Input: part model. Units: mm. Frame: model coordinates. Face numbers are marked on the shaded views. A direction names the side the tool comes from. Give positions to 0.01 mm unless a question says otherwise; leave off trailing zeros. Order: outer loops, then holes, each group sorted by start corner. A loop starts at its lowest first (then second) coordinate and runs counter-clockwise, first axis right, second up. Notation, with made-up numbers: (28, 4) - (67, 4) arc R21 ccw to (67, 28) - close; hole circle Ø9 at (35, 26.5). An arc over 180 degrees is marked (long way). Answer in a Markdown table with one row per item. Add a question column.
1. Mould query, pull axis X, two halves, no side actions, for the marked faces 1, 2, 3 and 4. Classes: released by +X, released by -X, zero draft, split by the parting line, or undercut.
2. Section query B-B on z = 7.5. Return loops of the section in (x, y) (3 decimals).
3. Section query C-C on z = -9. Return loops of the section in (x, y) (1 decimal).
4. Ray query, line 1 (Y direction, x = 17, z = 31); line 2 (X direction, y = -5.25, z = -25.5); line 3 (X direction, y = -3, z = -25). Return the intervals inside material, ascending. Write a range as [from, to].
5. Access query for the marked faces 5 and 6. Directions: +Z, -Z, +X, -X, +Y, -Y. A direction counts if a zero-diameter tool reaches every point of the face in a straight line with its end or side. Return the directions, or none.
6. Section query A-A on x = 12.7. Return loops of the section in (y, z) (1 decimal).
7. Contact query for flat-ended pins moving along their axis: pin 1 (6.5 mm diameter, centred on x = 37, y = -1, fed in from +Z); pin 2 (2 mm diameter, centred on y = -6, z = 27, fed in from +X); pin 3 (5 mm diameter, centred on x = 18.5, z = -7.5, fed in from +Y). Output: stop coordinate, or through.
```python
from build123d import *

# Parameters (mm, degrees)
EXTRUDE_THIN1_DEPTH = 38.1
EXTRUDE_THIN2_START = 12.7
EXTRUDE_THIN2_DEPTH = 12.7
REVOLVE_THIN1_ANGLE = 180
EXTRUDE_THIN3_START = -10.16
EXTRUDE_THIN3_DEPTH = 1.27


# Read off the part's stored shape, not the designer's step: Extrude-Thin3
with BuildPart() as part:
    # Sketch1 → Extrude-Thin1 (new body)
    with BuildSketch(Plane.XY):
        with BuildLine():
            ThreePointArc((-8.798818102, -5.08), (-5.08, -8.798818102), (0, -10.16))
            Line((0, -10.16), (25.4, -10.16))
            ThreePointArc((25.4, -10.16), (30.48, -8.798818102), (34.198818102, -5.08))
            Line((34.198818102, -5.08), (33.09896584, -4.445))
            ThreePointArc((33.09896584, -4.445), (29.845, -7.69896584), (25.4, -8.89))
            Line((25.4, -8.89), (0, -8.89))
            ThreePointArc((0, -8.89), (-4.445, -7.69896584), (-7.69896584, -4.445))
            Line((-7.69896584, -4.445), (-8.798818102, -5.08))
        make_face()
    extrude(amount=EXTRUDE_THIN1_DEPTH)

    # Sketch2 → Extrude-Thin2 (add)
    with BuildSketch(Plane(origin=(0, 0, 0), x_dir=(-1, 0, 0), z_dir=(0, 0, -1)).offset(EXTRUDE_THIN2_START)):
        with BuildLine():
            Line((-38.781535864, 2.8575), (-34.198818102, -5.08))
            ThreePointArc((-34.198818102, -5.08), (-30.48, -8.798818102), (-25.4, -10.16))
            Line((-25.4, -10.16), (0, -10.16))
            ThreePointArc((0, -10.16), (5.08, -8.798818102), (8.798818102, -5.08))
            Line((8.798818102, -5.08), (13.381535864, 2.8575))
            Line((13.381535864, 2.8575), (12.281683601, 3.4925))
            Line((12.281683601, 3.4925), (7.69896584, -4.445))
            ThreePointArc((7.69896584, -4.445), (4.445, -7.69896584), (0, -8.89))
            Line((0, -8.89), (-25.4, -8.89))
            ThreePointArc((-25.4, -8.89), (-29.845, -7.69896584), (-33.09896584, -4.445))
            Line((-33.09896584, -4.445), (-37.681683601, 3.4925))
            Line((-37.681683601, 3.4925), (-38.781535864, 2.8575))
        make_face()
    extrude(amount=-EXTRUDE_THIN2_DEPTH)

    # Sketch3 → Revolve-Thin1 (revolve)
    with BuildSketch(Plane(origin=(0, 0, -12.7), x_dir=(-1, 0, 0), z_dir=(0, 0, -1))):
        with BuildLine():
            ThreePointArc((0, -10.16), (5.08, -8.798818102), (8.798818102, -5.08))
            Line((8.798818102, -5.08), (13.381535864, 2.8575))
            Line((13.381535864, 2.8575), (12.281683601, 3.4925))
            Line((12.281683601, 3.4925), (7.69896584, -4.445))
            ThreePointArc((7.69896584, -4.445), (4.445, -7.69896584), (0, -8.89))
            Line((0, -8.89), (0, -10.16))
        make_face()
    revolve(axis=Axis((12.7, -10.16, -12.7), (0, -1, 0)), revolution_arc=REVOLVE_THIN1_ANGLE)

    # Extrude-Thin3 outline → Extrude-Thin3 (add)
    with BuildSketch(Plane(origin=(0, 0, 0), x_dir=(1, 0, 0), z_dir=(0, 1, 0)).offset(EXTRUDE_THIN3_START)):
        with BuildLine():
            Line((0, 12.7), (25.4, 12.7))
            ThreePointArc((25.4, 12.7), (12.7, 25.4), (0, 12.7))
        make_face()
    extrude(amount=EXTRUDE_THIN3_DEPTH)


solid = part.part
```
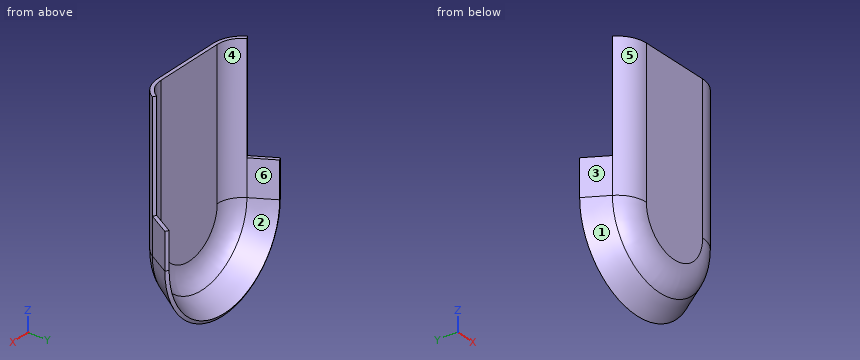
Answer:
| question | item | result |
|---|---|---|
| 1 | face 1 | split by the parting line |
| 1 | face 2 | undercut |
| 1 | face 3 | released by -X |
| 1 | face 4 | undercut |
| 2 | outline | (-8.799, -5.08) arc R10.16 ccw to (0, -10.16) - (25.4, -10.16) arc R10.16 ccw to (34.199, -5.08) - (33.099, -4.445) arc R8.89 cw to (25.4, -8.89) - (0, -8.89) arc R8.89 cw to (-7.699, -4.445) - close |
| 3 | outline | (-13.4, 2.9) - (-8.8, -5.1) arc R10.2 ccw to (0, -10.2) - (25.4, -10.2) arc R10.2 ccw to (34.2, -5.1) - (38.8, 2.9) - (37.7, 3.5) - (33.1, -4.4) arc R8.9 cw to (25.4, -8.9) - (0, -8.9) arc R8.9 cw to (-7.7, -4.4) - (-12.3, 3.5) - close |
| 4 | line 1 | y = [-10.16, -8.89] |
| 4 | line 2 | x = [-4.45, -2.5], [27.9, 29.85] |
| 4 | line 3 | x = [-6.38, -4.61], [30.01, 31.78] |
| 5 | face 5 | +Z, -Z, -X, -Y |
| 5 | face 6 | +Z, +Y |
| 6 | outline | (-10.2, -25.4) arc R10.2 ccw to (-5.1, -34.2) - (2.9, -38.8) - (3.5, -37.7) - (-4.4, -33.1) arc R8.9 cw to (-8.9, -25.4) - (-8.9, 38.1) - (-10.2, 38.1) - close |
| 7 | pin 1 | stops at z = 0 |
| 7 | pin 2 | stops at x = 34.2 |
| 7 | pin 3 | stops at y = -8.89 |
